from build123d import *

# Parameters (mm, degrees)
SK_PLACA_W                         = 220
SK_PLACA_H                         = 220
PLACA_DEPTH                        = 10
SK_PASO_CABLES_R                   = 30
PASO_CABLES_DEPTH                  = 10
SK_PASANTES_M4_PEDESTAL_R          = 2.25
PASANTES_M4_PEDESTAL_DEPTH         = 10
SK_CAJAS_M4_INFERIORES_R           = 4
CAJAS_M4_INFERIORES_DEPTH          = 4.5
SK_PASANTES_M4_SEPARADORES_CAJA_R  = 2.25
PASANTES_M4_SEPARADORES_CAJA_DEPTH = 10
SK_PASO_CABLES_CAJA_R              = 12.5
PASO_CABLES_CAJA_DEPTH             = 10
CROQUIS1_W                         = 40
CROQUIS1_H                         = 4
CROQUIS1_W_2                       = 4
CROQUIS1_H_2                       = 40
CORTAR_EXTRUIR1_DEPTH              = 156.884572681


with BuildPart() as part:
    # Sk_Placa → Placa (new body)
    with BuildSketch(Plane.XY):
        Rectangle(SK_PLACA_W, SK_PLACA_H)
    extrude(amount=PLACA_DEPTH)

    # Sk_Paso_cables → Paso_cables (cut)
    with BuildSketch(Plane.XY):
        Circle(SK_PASO_CABLES_R)
    extrude(amount=PASO_CABLES_DEPTH, mode=Mode.SUBTRACT)

    # Sk_Pasantes_M4_pedestal → Pasantes_M4_pedestal (cut)
    with BuildSketch(Plane.XY):
        with Locations((33.234018716, 33.234018716)):
            Circle(SK_PASANTES_M4_PEDESTAL_R)
        with Locations((-33.234018716, 33.234018716)):
            Circle(SK_PASANTES_M4_PEDESTAL_R)
        with Locations((-33.234018716, -33.234018716)):
            Circle(SK_PASANTES_M4_PEDESTAL_R)
        with Locations((33.234018716, -33.234018716)):
            Circle(SK_PASANTES_M4_PEDESTAL_R)
    extrude(amount=PASANTES_M4_PEDESTAL_DEPTH, mode=Mode.SUBTRACT)

    # Sk_Cajas_M4_inferiores → Cajas_M4_inferiores (cut)
    with BuildSketch(Plane.XY):
        with Locations((33.234018716, 33.234018716)):
            Circle(SK_CAJAS_M4_INFERIORES_R)
        with Locations((-33.234018716, 33.234018716)):
            Circle(SK_CAJAS_M4_INFERIORES_R)
        with Locations((-33.234018716, -33.234018716)):
            Circle(SK_CAJAS_M4_INFERIORES_R)
        with Locations((33.234018716, -33.234018716)):
            Circle(SK_CAJAS_M4_INFERIORES_R)
    extrude(amount=CAJAS_M4_INFERIORES_DEPTH, mode=Mode.SUBTRACT)

    # Sk_Pasantes_M4_separadores_caja → Pasantes_M4_separadores_caja (cut)
    with BuildSketch(Plane.XY):
        with Locations((-95, -95)):
            Circle(SK_PASANTES_M4_SEPARADORES_CAJA_R)
        with Locations((-95, 95)):
            Circle(SK_PASANTES_M4_SEPARADORES_CAJA_R)
        with Locations((95, -95)):
            Circle(SK_PASANTES_M4_SEPARADORES_CAJA_R)
        with Locations((95, 95)):
            Circle(SK_PASANTES_M4_SEPARADORES_CAJA_R)
    extrude(amount=PASANTES_M4_SEPARADORES_CAJA_DEPTH, mode=Mode.SUBTRACT)

    # Sk_Paso_cables_caja → Paso_cables_caja (cut)
    with BuildSketch(Plane.XY):
        with Locations((-60, -70)):
            Circle(SK_PASO_CABLES_CAJA_R)
    extrude(amount=PASO_CABLES_CAJA_DEPTH, mode=Mode.SUBTRACT)

    # Croquis1 → Cortar-Extruir1 (cut, through all)
    with BuildSketch(Plane.XY.offset(10)):
        with Locations((0, -95)):
            Rectangle(CROQUIS1_W, CROQUIS1_H)
        with Locations((0, 95)):
            Rectangle(CROQUIS1_W, CROQUIS1_H)
        with Locations((93, 0)):
            Rectangle(CROQUIS1_W_2, CROQUIS1_H_2)
        with Locations((-93, 0)):
            Rectangle(CROQUIS1_W_2, CROQUIS1_H_2)
    extrude(amount=-CORTAR_EXTRUIR1_DEPTH, mode=Mode.SUBTRACT)


solid = part.part
CAD build for the part. Positions are in the model's coordinates, mm. A direction names the side the tool comes from. Coordinates: 2 decimals unless noted, no trailing zeros. Loops run counter-clockwise (first coordinate to the right, second up) from the corner with the lowest first, then second, coordinate; pieces in that order, holes last. Notation, with made-up numbers: (-19, 65.5) - (26, 65.5) arc R31 cw to (26, 97.5) - close; hole circle Ø10 at (44, 72). An arc over 180 degrees is marked (long way). Use one line per item in the form item = value. Start each with the question number.
1) Band-saw the part on D-D (z = 3). State how many separate pieces and enclosed holes the cut face has, and give its area (3 significant figures).
2) Band-saw the part on A-A (y = -70). Give the cut face in (x, z), and give its area (3 significant figures).
3) Band-saw the part on C-C (x = -59). Give the cut face in (y, z), and give its area (3 significant figures).
4) Drill centre lines: L1, parallel to X at y = -96, z = 3.75; L2, parallel to Y at x = 0, z = 5; L3, parallel to X at y = -5, z = 4.75. Where is each one in solid material? Low to high. Write a range as from..to.
5) Flat gauge pins, fed straight in: pin 1 (5 mm diameter, centred on x = -33.23, y = -33.23, fed in from -Z); pin 2 (4 mm diameter, centred on x = -95, y = -95, fed in from -Z). Where does each tip first touch, or does it go through?
6) Two-plate mould, pull along X, no slides. Class faces 4 (the face through (0, -97, 5)), 5 (the face through (-26, 26, 10)), 6 (the face through (110, -2, 5)): +X half, -X half, draft (parallel to the pull), parting line (faces both ways), or undercut.
7) Band-saw the part on B-B (y = 0). Give the cut face in (x, z), and give its area (3 significant figures).
8) Tool access for faces 1 (the face through (-26, 26, 0)), 2 (the face through (35.08, -36.783, 2.218)), 3 (the face through (91, 0, 5)): list every direction of +Z, -Z, +X, -X, +Y, -Y with a clear straight run to the whole face (end or side of a thin tool).
Check values:
q1.separate_pieces = 1
q1.enclosed_holes = 14
q1.area = 44,200 mm2
q2.outline = (-110, 0) - (-72.5, 0) - (-72.5, 10) - (-110, 10) - close; (-47.5, 0) - (110, 0) - (110, 10) - (-47.5, 10) - close
q2.area = 1,950 mm2
q3.outline = (-110, 0) - (-82.46, 0) - (-82.46, 10) - (-110, 10) - close; (-57.54, 0) - (110, 0) - (110, 10) - (-57.54, 10) - close
q3.area = 1,950 mm2
q4.L1 = -110..-97.02, -92.98..-20, 20..92.98, 97.02..110
q4.L2 = -110..-97, -93..-30, 30..93, 97..110
q4.L3 = -110..-95, -91..-29.58, 29.58..91, 95..110
q5.pin_1 = 4.5
q5.pin_2 = through
q6.face_4 = undercut
q6.face_5 = draft
q6.face_6 = +X half
q7.outline = (-110, 0) - (-95, 0) - (-95, 10) - (-110, 10) - close; (-91, 0) - (-30, 0) - (-30, 10) - (-91, 10) - close; (30, 0) - (91, 0) - (91, 10) - (30, 10) - close; (95, 0) - (110, 0) - (110, 10) - (95, 10) - close
q7.area = 1,520 mm2
q8.face_1 = -Z, +X, -X, +Y, -Y
q8.face_2 = -Z
q8.face_3 = +Z, -Z
